```python
from build123d import *

# Parameters (mm, degrees)
SKETCH_1_W          = 29.6
SKETCH_1_H          = 59.6
SKETCH_1_W_2        = 5
SKETCH_1_H_2        = 30
EXTRUDE_1_DEPTH     = 20
SKETCH_2_W          = 39.6
SKETCH_2_H          = 69.6
SKETCH_2_W_2        = 5
SKETCH_2_H_2        = 30
EXTRUDE_2_DEPTH     = 3
SKETCH_3_W          = 4.5
SKETCH_3_H          = 6.4
CUT_EXTRUDE_1_DEPTH = 11
SKETCH_5_W          = 6.4
SKETCH_5_H          = 6
CUT_EXTRUDE_2_DEPTH = 35.6


with BuildPart() as part:
    # 스케치1 → 보스-돌출1 (new body)
    with BuildSketch(Plane.XY):
        Rectangle(SKETCH_1_W, SKETCH_1_H)
        with Locations((0, 9.8)):
            Rectangle(SKETCH_1_W_2, SKETCH_1_H_2, mode=Mode.SUBTRACT)
    extrude(amount=EXTRUDE_1_DEPTH)

    # 스케치2 → 보스-돌출2 (add)
    with BuildSketch(Plane(origin=(0, 0, 0), x_dir=(-1, 0, 0), z_dir=(0, 0, -1))):
        Rectangle(SKETCH_2_W, SKETCH_2_H)
        with Locations((0, 9.8)):
            Rectangle(SKETCH_2_W_2, SKETCH_2_H_2, mode=Mode.SUBTRACT)
    extrude(amount=EXTRUDE_2_DEPTH)

    # 스케치3 → 컷-돌출1 (cut)
    with BuildSketch(Plane(origin=(0, 29.8, 0), x_dir=(1, 0, 0), z_dir=(0, 1, 0))):
        with Locations((-7.05, -10)):
            Rectangle(SKETCH_3_W, SKETCH_3_H)
        with Locations((7.05, -10)):
            Rectangle(SKETCH_3_W, SKETCH_3_H)
    extrude(amount=-CUT_EXTRUDE_1_DEPTH, mode=Mode.SUBTRACT)

    # 스케치5 → 컷-돌출2 (cut, through all)
    with BuildSketch(Plane.ZY.offset(14.8)):
        with Locations((10, 21.8)):
            Rectangle(SKETCH_5_W, SKETCH_5_H)
    extrude(amount=-CUT_EXTRUDE_2_DEPTH, mode=Mode.SUBTRACT)


solid = part.part
```
Verification items for the finished model (mm, model axes). A direction names the side the tool comes from. Round coordinates to 2 decimals unless told otherwise and drop trailing zeros. Write each loop counter-clockwise with the first axis right and the second up, starting at its lowest first coordinate (ties: lowest second). Pieces come first, ordered by that corner, then holes. Notation, with made-up numbers: (-29.75, -36.75) -> (4.25, -36.75) arc R23 ccw to (4.25, 1.25) -> close; hole circle Ø5 at (-5, -34). An arc over 180 degrees is marked (long way). Write each question's results on one line, items separated by ' | '.
Q1. Thickness scan on probe 1 along X at (y, z) = (27, 9.25); probe 2 along X at (y, z) = (-3, 7.5); probe 3 along Y at (x, z) = (4.5, 8). Record the ranges inside material, lowest first.
Derived:
probe 1: x = -14.8 to -9.3, -4.8 to 4.8, 9.3 to 14.8 | probe 2: x = -14.8 to -2.5, 2.5 to 14.8 | probe 3: y = -29.8 to 18.8, 24.8 to 29.8
Q2. Sectioned sample at C-C, the plane z = 1. Record the boundary of the cut face in (x, y), and give its area (3 significant figures).
Derived:
outline: (-14.8, -29.8) -> (14.8, -29.8) -> (14.8, 29.8) -> (-14.8, 29.8) -> close; hole (-2.5, -5.2) -> (2.5, -5.2) -> (2.5, 24.8) -> (-2.5, 24.8) -> close | area: 1,610 mm²
Q3. Sectioned sample at A-A, the plane z = 10.75. Record the boundary of the cut face in (x, y).
Derived:
outline: (-14.8, -29.8) -> (14.8, -29.8) -> (14.8, 18.8) -> (2.5, 18.8) -> (2.5, -5.2) -> (-2.5, -5.2) -> (-2.5, 18.8) -> (-14.8, 18.8) -> close; (-14.8, 24.8) -> (-9.3, 24.8) -> (-9.3, 29.8) -> (-14.8, 29.8) -> close; (-4.8, 24.8) -> (4.8, 24.8) -> (4.8, 29.8) -> (-4.8, 29.8) -> close; (9.3, 24.8) -> (14.8, 24.8) -> (14.8, 29.8) -> (9.3, 29.8) -> close
Q4. Access from +Z, -Z, +X, -X, +Y, -Y to the whole of each face (thin tool, end or side, straight path). Record for faces 4 (the face through (9.3, 27, 10)), 5 (the face through (9, 18.8, 10)), 6 (the face through (14.8, 0, 10)), 7 (the face through (-9, 23, 6.8)).
Derived:
face 4: +Y | face 5: +X, -X | face 6: +Z, +X, +Y, -Y | face 7: none
Q5. Go/stop test with flat-tipped pins: pin 1 Ø5.5 at (y, z) = (27.5, 11) entering from +X; pin 2 Ø10 at (y, z) = (17.5, 14) entering from -X; pin 3 Ø3 at (x, z) = (-7.5, 14.5) entering from +Y. Record where each tip stops, or that it passes through.
Derived:
pin 1: stops at x = 14.8 | pin 2: stops at x = -14.8 | pin 3: stops at y = 29.8
Q6. Sectioned sample at B-B, the plane y = 27. Record the boundary of the cut face in (x, z), and give its area (3 significant figures).
Derived:
outline: (-19.8, -3) -> (19.8, -3) -> (19.8, 0) -> (14.8, 0) -> (14.8, 20) -> (-14.8, 20) -> (-14.8, 0) -> (-19.8, 0) -> close; hole (-9.3, 6.8) -> (-4.8, 6.8) -> (-4.8, 13.2) -> (-9.3, 13.2) -> close; hole (4.8, 6.8) -> (9.3, 6.8) -> (9.3, 13.2) -> (4.8, 13.2) -> close | area: 653 mm²
Q7. Draft check along X on faces 1 (the face through (19.8, 0, -1)), 2 (the face through (-4.8, 27, 10)), 3 (the face through (12, 24.8, 10)). Enter one of: released by +X, released by -X, zero draft, split by the parting line, or undercut.
Derived:
face 1: released by +X | face 2: undercut | face 3: zero draft
Q8. Sectioned sample at D-D, the plane y = 2. Record the boundary of the cut face in (x, z).
Derived:
outline: (-19.8, -3) -> (-2.5, -3) -> (-2.5, 20) -> (-14.8, 20) -> (-14.8, 0) -> (-19.8, 0) -> close; (2.5, -3) -> (19.8, -3) -> (19.8, 0) -> (14.8, 0) -> (14.8, 20) -> (2.5, 20) -> close
